Autodesk Inventor part; units mm, degrees
ref_plane "YZ Plane" through (0, 0, 0) normal (1, 0, 0) x (0, 1, 0)
ref_plane "XZ Plane" through (0, 0, 0) normal (0, 1, 0) x (-1, 0, 0)
ref_plane "XY Plane" through (0, 0, 0) normal (0, 0, 1) x (1, 0, 0)
sketch "Эскиз2" plane through (0, 0, 0) normal (0, 1, 0) x (-1, 0, 0)
  line L0 (0, 0) -> (10, 0)
  line L1 (10, 0) -> (10, -1.7)
  line L2 (10, -1.7) -> (1.2, -1.7)
  line L3 (1.2, -1.7) -> (1.2, -13.5)
  line L4 (1.2, -13.5) -> (10, -13.5)
  line L5 (10, -13.5) -> (10, -15.2)
  line L6 (10, -15.2) -> (0, -15.2)
  line L7 (0, -15.2) -> (0, 0)
  dimension "d0" = 10
  dimension "d1" = 1.7
  dimension "d4" = 1.7
  dimension "d5" = 1.2
  dimension "d10" = 15.2
extrude "Выдавливание1" add sketch "Эскиз2" along normal blind 50
fillet "Сопряжение1" radius 2 4 edges at (-10, 50, -14.35) (-10, 50, -0.85) (-10, 0, -14.35) (-10, 0, -0.85)
sketch "Эскиз3" plane through (0, 0, 0) normal (1, 0, 0) x (0, 0, -1)
  line L0 (13.5, 0) -> (1.7, 0)
  line L1 (5.5, 0) -> (7.5, 20)
  line L2 (7.5, 20) -> (9.5, 0)
  line L3 (9.5, 0) -> (5.5, 0)
  line L4 (13.5, 50) -> (1.7, 50)
  line L5 (5.5, 50) -> (7.5, 30)
  line L6 (7.5, 30) -> (9.5, 50)
  line L7 (9.5, 50) -> (5.5, 50)
  line L8 (0, 0) -> (0, 50)
  point P0 (7.6, 50)
  point P1 (7.5, 0)
  point P2 (7.5, 50)
  point P3 (9.5, 0)
  dimension "d11" = 20
  dimension "d12" = 20
  dimension "d15" = 0
  dimension "d16" = 0
  dimension "d17" = 7.5
  dimension "d18" = 7.5
  dimension "d19" = 4
  dimension "d20" = 4
extrude "Выдавливание2" cut sketch "Эскиз3" against normal blind 10
fillet "Сопряжение3" radius 2 4 edges at (-0.6, 0, -9.5) (-0.6, 0, -5.5) (-0.6, 50, -5.5) (-0.6, 50, -9.5)
fillet "Сопряжение4" radius 0.1 47 edges at (-9.4142, 49.4142, -15.2) (-4, 50, -15.2) (-9.4142, 0.5858, -15.2) (-4, 0, -15.2) (-10, 25, -15.2) (-9.4142, 49.4142, -13.5) (-4.6, 50, -13.5) (-9.4142, 0.5858, -13.5) (-4.6, 0, -13.5) (-10, 25, -13.5) (-1.2, 25, -13.5) (-1.2, 49.4829, -9.968) (-1.2, 50, -12.405) (-1.2, 39.0995, -8.41) (-1.2, 49.4829, -5.032) (-1.2, 50, -2.695) (-1.2, 39.0995, -6.59) (0, 49.4829, -5.032) (0, 50, -1.845) (0, 39.0995, -6.59) (0, 49.4829, -9.968) (0, 50, -13.255) (0, 39.0995, -8.41) (-1.2, 0.5171, -9.968) (-1.2, 0, -12.405) (-1.2, 10.9005, -8.41) (0, 0.5171, -9.968) (0, 0, -13.255) (0, 10.9005, -8.41) (-1.2, 0.5171, -5.032) (-1.2, 0, -2.695) (-1.2, 10.9005, -6.59) (0, 0.5171, -5.032) (0, 0, -1.845) (0, 10.9005, -6.59) (-9.4142, 49.4142, -1.7) (-4.6, 50, -1.7) (-9.4142, 0.5858, -1.7) (-4.6, 0, -1.7) (-10, 25, -1.7) (-9.4142, 49.4142, 0) (-4, 50, 0) (-9.4142, 0.5858, 0) (-4, 0, 0) (-10, 25, 0) (0, 25, 0) (0, 25, -15.2)
properties part number "Соединитель"
Geometry: final body of the model. Coordinates: model frame, mm. A direction names the side the tool comes from. Coordinates: 2 decimals unless noted, no trailing zeros. Order: outer loops, then holes, each group sorted by start corner. A loop starts at its lowest first (then second) coordinate and runs counter-clockwise, first axis right, second up. Notation, with made-up numbers: (-7.75, -12.75) - (4.25, -12.75) arc R29 ccw to (4.25, 16.25) - close; hole circle Ø7 at (-27.5, 51). An arc over 180 degrees is marked (long way). Use one line per item in the form item = value.
1) Section B-B (z = -2.25). Return loops of the section in (x, y), then the cut area to 3 significant figures.
Solutions:
outline = (-1.2, 0.1) arc R0.1 ccw to (-1.1, 0) - (-0.1, 0) arc R0.1 ccw to (0, 0.1) - (0, 49.9) arc R0.1 ccw to (-0.1, 50) - (-1.1, 50) arc R0.1 ccw to (-1.2, 49.9) - close
area = 60.0 mm^2
2) Mould query, pull axis Z, two halves, no side actions, for faces 6 (the face through (-9.43, 49.4, -0.86)), 7 (the face through (-0.607, 49.497, -5.017)). Classes: +Z half, -Z half, draft (parallel to the pull), parting line (faces both ways), or undercut.
Solutions:
face_6 = draft
face_7 = undercut
3) Set-up query: faces 1 (the face through (-0.593, 39.227, -6.577)), 2 (the face through (-0.607, 0.531, -5.047)), 3 (the face through (-4, 0, -1)), 4 (the face through (-1.2, 25, -7)), 5 (the face through (-9.43, 49.4, -14.36)). Return all of +Z, -Z, +X, -X, +Y, -Y with unobstructed straight access to the full face (end or side cutting, diameter ignored); none if empty.
Solutions:
face_1 = +X, -X, +Y
face_2 = +X, -X, -Y
face_3 = +Z, -Z, +X, -X, -Y
face_4 = -X, +Y, -Y
face_5 = +Z, -Z, -X, +Y
4) Ray query, L1, parallel to Z at x = -1.75, y = 8; L2, parallel to X at y = 20, z = -6.75; L3, parallel to Z at x = -1, y = 16. Return the intervals inside material, ascending.
Solutions:
L1 = -15.2 to -13.5, -1.7 to 0
L2 = -1.2 to 0
L3 = -15.2 to -7.9, -7.1 to 0
5) Section A-A (x = -7.25). Return loops of the section in (y, z), then the cut area to 3 significant figures.
Solutions:
outline = (0, -15.1) arc R0.1 ccw to (0.1, -15.2) - (49.9, -15.2) arc R0.1 ccw to (50, -15.1) - (50, -13.6) arc R0.1 ccw to (49.9, -13.5) - (0.1, -13.5) arc R0.1 ccw to (0, -13.6) - close; (0, -1.6) arc R0.1 ccw to (0.1, -1.7) - (49.9, -1.7) arc R0.1 ccw to (50, -1.6) - (50, -0.1) arc R0.1 ccw to (49.9, 0) - (0.1, 0) arc R0.1 ccw to (0, -0.1) - close
area = 170 mm^2
